Model file for the job. Use its own axes, mm. A direction names the side the tool comes from. Round coordinates to 2 decimals unless told otherwise and drop trailing zeros. Order: outer loops, then holes, each group sorted by start corner. A loop starts at its lowest first (then second) coordinate and runs counter-clockwise, first axis right, second up. Notation, with made-up numbers: (7.25, 87) - (51.25, 87) arc R27 ccw to (51.25, 115) - close; hole circle Ø10 at (51.25, -7). An arc over 180 degrees is marked (long way). Write item = value, one per line.
Autodesk Inventor part; units mm, degrees
ref_plane "YZ Plane" through (0, 0, 0) normal (1, 0, 0) x (0, 1, 0)
ref_plane "XZ Plane" through (0, 0, 0) normal (0, 1, 0) x (-1, 0, 0)
ref_plane "XY Plane" through (0, 0, 0) normal (0, 0, 1) x (1, 0, 0)
sketch "Sketch1" plane through (0, 0, 0) normal (0, 1, 0) x (-1, 0, 0)
  line L0 (-13, -11.9282) -> (10, -11.9282)
  line L1 (10, -11.9282) -> (10, 11.9282)
  line L2 (10, 11.9282) -> (-13, 11.9282)
  line L3 (-13, 11.9282) -> (-13, -11.9282)
  circle A0 centre (-8, 0) radius 4
  circle A1 centre (4, -6.9282) radius 4
  circle A2 centre (4, 6.9282) radius 4
  circle A3 centre (0, 0) radius 8 construction
  circle A4 centre (0, 0) radius 1.75
  dimension "d11" = 16
  dimension "d2" = 8
  dimension "d6" = 360
  dimension "d8" = 6
  dimension "d9" = 5
  dimension "d12" = 5
  dimension "d13" = 5
  dimension "d35" = 3.5
extrude "Extrusion1" add sketch "Sketch1" along normal blind 3
sketch "Sketch2" plane through (0, 3, 0) normal (0, 1, 0) x (1, 0, 0)
  circle A0 centre (-4, -6.9282) radius 4
  circle A1 centre (-4, 6.9282) radius 4
  circle A2 centre (8, 0) radius 4
  line L0 (13, 11.9282) -> (-10, 11.9282)
  line L1 (-10, 11.9282) -> (-10, -11.9282)
  line L2 (-10, -11.9282) -> (13, -11.9282)
  line L3 (13, -11.9282) -> (13, 11.9282)
  circle A3 centre (0, 0) radius 1.75
  dimension "d16" = 3.5
extrude "Extrusion2" add sketch "Sketch2" along normal blind 1.5 contours A0 | A1 | A2 | L3 L2 L1 L0
sketch "Sketch3" plane through (0, 0, 0) normal (0, -1, 0) x (1, 0, 0)
  circle A0 centre (-4, 6.9282) radius 4
  circle A1 centre (-4, -6.9282) radius 4
  circle A2 centre (8, 0) radius 4
  line L0 (13, -11.9282) -> (-10, -11.9282)
  line L1 (13, 11.9282) -> (13, -11.9282)
  line L2 (-10, 11.9282) -> (13, 11.9282)
  line L3 (-10, -11.9282) -> (-10, 11.9282) construction
  line L4 (-2, 11.9282) -> (13, 2.9282)
  line L5 (13, 11.9282) -> (13, -11.9282)
  line L6 (13, -2.9282) -> (-2, -11.9282)
  point P0 (0, 0)
  dimension "d19" = 9
  dimension "d20" = 9
  dimension "d21" = 15
  dimension "d22" = 15
extrude "Extrusion3" cut sketch "Sketch3" against normal through all contours L4 L2 L1 | L0 L6 L1
sketch "Sketch5" plane through (0, 0, 0) normal (0, -1, 0) x (1, 0, 0)
  line L0 (13, 2.9282) -> (-2, 11.9282)
  line L1 (-10, 11.9282) -> (-2, 11.9282)
  line L2 (-10, -11.9282) -> (-10, 11.9282)
  line L3 (-2, -11.9282) -> (-10, -11.9282)
  line L4 (-2, -11.9282) -> (13, -2.9282)
  line L5 (13, 2.9282) -> (13, -2.9282)
  circle A0 centre (-4, 6.9282) radius 4
  circle A1 centre (-4, -6.9282) radius 4
  circle A2 centre (8, 0) radius 4
  line L6 (17, -5.193) -> (-0.8921, -15.9282)
  line L7 (-0.8921, -15.9282) -> (-14, -15.9282)
  line L8 (-14, -15.9282) -> (-14, 15.9282)
  line L9 (-14, 15.9282) -> (-0.8921, 15.9282)
  line L10 (-0.8921, 15.9282) -> (17, 5.193)
  line L11 (17, 5.193) -> (17, -5.193)
  line L12 (13, -2.9282) -> (13, -7.593)
  line L13 (13, 2.8448) -> (13, 7.593)
  line L14 (-2, -11.9282) -> (-10, -11.9282)
  line L15 (-10, -11.9282) -> (-10, -15.9282)
  line L16 (-10, 11.9282) -> (-2, 11.9282)
  line L17 (-10, 11.9282) -> (-10, 15.9282)
  line L18 (-2, -11.9282) -> (13, -2.9282)
  line L19 (13, -2.9282) -> (-2, -11.9282)
  line L20 (-2, -11.9282) -> (-10, -11.9282)
  line L21 (-10, -11.9282) -> (-10, 11.9282)
  line L22 (-10, 11.9282) -> (-2, 11.9282)
  line L23 (13, 2.9282) -> (-2, 11.9282)
  line L24 (13, 2.9282) -> (-2, 11.9282)
  line L25 (13, -2.9282) -> (13, 2.8448)
  point P0 (0, 0)
  dimension "d27" = 4
extrude "Extrusion5" add sketch "Sketch5" against normal up to surface (4.5 mm away) contours L0 L1 L17 L9 L10 L13 | L12 L6 L7 L15 L3 L4
sketch "Sketch6" plane through (0, 4.5, 0) normal (0, 1, 0) x (1, 0, 0)
  line L0 (13, -7.593) -> (13, 7.593)
  line L1 (-0.8921, 15.9282) -> (13, 7.593)
  line L2 (-10, 15.9282) -> (-0.8921, 15.9282)
  line L3 (-10, -15.9282) -> (-10, 15.9282)
  line L4 (-0.8921, -15.9282) -> (-10, -15.9282)
  line L5 (13, -7.593) -> (-0.8921, -15.9282)
  line L6 (13, 7.593) -> (-0.8921, 15.9282)
  line L7 (-0.8921, 15.9282) -> (-2.4356, 13.3557)
  line L8 (-2.4356, 13.3557) -> (11.4565, 5.0205)
  line L9 (11.4565, 5.0205) -> (13, 7.593)
  line L10 (13, -7.593) -> (13, 7.593)
  line L11 (13, -7.593) -> (-0.8921, -15.9282)
  line L12 (-0.8921, -15.9282) -> (-2.4356, -13.3557)
  line L13 (-2.4356, -13.3557) -> (11.4565, -5.0205)
  line L14 (11.4565, -5.0205) -> (13, -7.593)
  point P0 (0, 0)
  dimension "d30" = 3
  dimension "d31" = 3
extrude "Extrusion6" [suppressed]
sketch "Sketch7" plane through (0, 4.5, 0) normal (0, 1, 0) x (1, 0, 0)
  line L0 (13, -7.593) -> (13, 7.593)
  line L1 (-0.8921, 15.9282) -> (13, 7.593)
  line L2 (-10, 15.9282) -> (-0.8921, 15.9282)
  line L3 (-10, -15.9282) -> (-10, 15.9282)
  line L4 (-0.8921, -15.9282) -> (-10, -15.9282)
  line L5 (13, -7.593) -> (-0.8921, -15.9282)
  circle A0 centre (0, 0) radius 1.75
  line L6 (1.6166, 2.8) -> (3.2332, 0)
  line L7 (3.2332, 0) -> (1.6166, -2.8)
  line L8 (1.6166, -2.8) -> (-1.6166, -2.8)
  line L9 (-1.6166, -2.8) -> (-3.2332, 0)
  line L10 (-3.2332, 0) -> (-1.6166, 2.8)
  line L11 (-1.6166, 2.8) -> (1.6166, 2.8)
  line L12 (-1.6166, 2.8) -> (-11.6048, 2.8)
  line L13 (-11.6048, 2.8) -> (-11.6048, -2.8)
  line L14 (-11.6048, -2.8) -> (-1.6166, -2.8)
  line L15 (-1.6166, -2.8) -> (-1.6166, 2.8)
  dimension "d39" = 5.6
extrude "Extrusion7" cut sketch "Sketch7" against normal blind 3.5 contours L14 L13 L12 L3 | L3 L12 L10 L9 L14 | L15 A0 L11 L6 L7 L8 | L9 L10 L15 A0
sketch "Sketch8" plane through (0, 4.5, 0) normal (0, 1, 0) x (1, 0, 0)
  line L0 (-10, 2.8) -> (1.6166, 2.8)
  line L1 (1.6166, 2.8) -> (3.2332, 0)
  line L2 (3.2332, 0) -> (1.6166, -2.8)
  line L3 (1.6166, -2.8) -> (-10, -2.8)
  line L4 (-10, -15.9282) -> (-10, -2.8)
  line L5 (-0.8921, -15.9282) -> (-10, -15.9282)
  line L6 (13, -7.593) -> (-0.8921, -15.9282)
  line L7 (13, -7.593) -> (13, 7.593)
  line L8 (-0.8921, 15.9282) -> (13, 7.593)
  line L9 (-10, 15.9282) -> (-0.8921, 15.9282)
  line L10 (-10, 2.8) -> (-10, 15.9282)
  line L11 (-10, 2.8) -> (-10, 15.9282)
  line L12 (-10, -15.9282) -> (-10, -2.8)
  line L13 (-10, 2.8) -> (-10, -2.8)
  circle A0 centre (0, 0) radius 1.75
extrude "Extrusion8" add sketch "Sketch8" along normal blind 1
equation "\"d12\" = d9"
equation "\"d13\" = d9"
properties part number "30_Cube_Z_Focus_Drylin_NEMA_slide_part1"
1) Cut at A-A (y = 5). Write the cut outline in (x, z).
Conclusion:
outline = (-10, -15.93) - (-0.89, -15.93) - (13, -7.59) - (13, 7.59) - (-0.89, 15.93) - (-10, 15.93) - close; hole circle Ø3.5 at (0, 0)
2) Cut at B-B (x = -4). Write the cut outline in (y, z).
Conclusion:
outline = (0, -15.93) - (5.5, -15.93) - (5.5, 15.93) - (0, 15.93) - (0, 10.93) - (3, 10.93) - (3, 2.93) - (0, 2.93) - (0, -2.93) - (3, -2.93) - (3, -10.93) - (0, -10.93) - close; hole (1, -2.8) - (4.5, -2.8) - (4.5, 2.8) - (1, 2.8) - close
3) Cut at D-D (y = 2.2). Write the cut outline in (x, z).
Conclusion:
outline = (-10, -15.93) - (-0.89, -15.93) - (13, -7.59) - (13, 7.59) - (-0.89, 15.93) - (-10, 15.93) - (-10, 2.8) - (1.62, 2.8) - (3.23, 0) - (1.62, -2.8) - (-10, -2.8) - close; hole circle Ø8 at (-4, -6.93); hole circle Ø8 at (-4, 6.93); hole circle Ø8 at (8, 0)
4) 3-axis set-ups, long thin cutter, end or side, ignore diameter. For faces 4 (the face through (-4, 3, 7)), 5 (the face through (-4.1, 3.2, -2.8)), 6 (the face through (1, 5.5, -4)): which of +Z, -Z, +X, -X, +Y, -Y reach the whole face in a straight line?
Conclusion:
face_4 = -Y
face_5 = -X
face_6 = +Z, -Z, +X, -X, +Y
5) Cut at C-C (z = 1). Write the cut outline in (x, y).
Conclusion:
outline = (-10, 0) - (-1.44, 0) - (-1.44, 1) - (-10, 1) - close; (-10, 4.5) - (-1.44, 4.5) - (-1.44, 5.5) - (-10, 5.5) - close; (1.44, 0) - (4.13, 0) - (4.13, 3) - (11.87, 3) - (11.87, 0) - (13, 0) - (13, 5.5) - (1.44, 5.5) - (1.44, 4.5) - (2.66, 4.5) - (2.66, 1) - (1.44, 1) - close
6) Flat gauge pins, fed straight in: pin 1 Ø3 at (y, z) = (2, 12.5) entering from +X; pin 2 Ø4 at (x, z) = (-5, 5.5) entering from -Y; pin 3 Ø2 at (x, z) = (0, 0) entering from -Y; pin 4 Ø1.5 at (x, y) = (3.5, 2.5) entering from +Z. Where does each tip first touch, or does it go through?
Conclusion:
pin_1 = 7.32
pin_2 = 3
pin_3 = through
pin_4 = 13.74
7) Mould opens along Y. For faces 1 (the face through (8, 3, 0)), 2 (the face through (-5, 1, 0)), 3 (the face through (-5, 3, -15.928)) say: +Y half, -Y half, draft (parallel to the pull), parting line (faces both ways), or undercut.
Conclusion:
face_1 = -Y half
face_2 = undercut
face_3 = draft
8) Wall check: line 1 along Z through (x, y) = (-4, 0.95); line 2 along Z through (x, y) = (-3.5, 0.5); line 3 along Z through (x, y) = (-7.25, 3.1). Give the ranges that are in metal, low to high.
Conclusion:
line_1 = -15.93 to -10.93, -2.93 to 2.93, 10.93 to 15.93
line_2 = -15.93 to -10.9, -2.96 to 2.96, 10.9 to 15.93
line_3 = -15.93 to -2.8, 2.8 to 15.93
